```python
from build123d import *

# Parameters (mm, degrees)
SKETCH1_R           = 2.1
BOSS_EXTRUDE1_DEPTH = 200


with BuildPart() as part:
    # Sketch1 → Boss-Extrude1 (new body)
    with BuildSketch(Plane(origin=(0, 0, 0), x_dir=(1, 0, 0), z_dir=(0, 1, 0))):
        Polygon((1.8, 15.5), (1.8, 13.1), (0, 14.9), (0, 20), (5.1, 20), (6.9, 18.2), (4.5, 18.2), (4.5, 16.560660172), (7.190031555, 13.870628617), (12.839339828, 13.870628617), (15.529414018, 16.560702806), (15.529414018, 18.2), (13.1, 18.2), (14.9, 20), (25.280697212, 20), (27.080697212, 18.2), (24.470585982, 18.2), (24.470585982, 16.560702806), (27.160660172, 13.870628617), (32.809968445, 13.870628617), (35.5, 16.560660172), (35.5, 18.2), (33.1, 18.2), (34.9, 20), (40, 20), (40, 14.9), (38.2, 13.1), (38.2, 15.5), (36.560660172, 15.5), (33.870585982, 12.809925811), (33.870585982, 7.160617537), (36.560617537, 4.470585982), (38.2, 4.470585982), (38.2, 6.9), (40, 5.1), (40, 0), (34.9, 0), (33.1, 1.8), (35.499957366, 1.8), (35.499957366, 3.409925811), (32.809883176, 6.1), (27.160574903, 6.1), (24.470543348, 3.409968445), (24.470543348, 1.8), (27, 1.8), (25.2, 0), (14.9, 0), (13.1, 1.8), (15.529456652, 1.8), (15.529456652, 3.409968445), (12.839425097, 6.1), (7.190116824, 6.1), (4.500042634, 3.409925811), (4.500042634, 1.8), (6.9, 1.8), (5.1, 0), (0, 0), (0, 5.1), (1.8, 6.9), (1.8, 4.470585982), (3.439382463, 4.470585982), (6.129414018, 7.160617537), (6.129414018, 12.809925811), (3.439339828, 15.5), align=None)
        with Locations(Location((10, 10, 0), (0, 0, 270))):
            Circle(SKETCH1_R, mode=Mode.SUBTRACT)
        with Locations(Location((30, 10, 0), (0, 0, 90))):
            Circle(SKETCH1_R, mode=Mode.SUBTRACT)
        Polygon((13.900042634, 7.175345863), (13.900042634, 12.824654137), (17.029456652, 15.964292458), (17.039482597, 18.2), (22.960517403, 18.2), (22.970543348, 15.964292458), (26.099957366, 12.824654137), (26.099957366, 7.175345863), (22.970543348, 4.035707542), (22.970543348, 1.8), (17.029456652, 1.8), (17.029456652, 4.035707542), align=None, mode=Mode.SUBTRACT)
    extrude(amount=BOSS_EXTRUDE1_DEPTH)


solid = part.part
```
Model file for the job. Use its own axes, mm. A direction names the side the tool comes from. Give positions to 0.01 mm unless a question says otherwise; leave off trailing zeros. Write each loop counter-clockwise with the first axis right and the second up, starting at its lowest first coordinate (ties: lowest second). Pieces come first, ordered by that corner, then holes. Notation, with made-up numbers: (76, 15.25) - (92, 15.25) arc R27 cw to (92, 31.25) - close; hole circle Ø9 at (-17, -16.75). An arc over 180 degrees is marked (long way). One line per question, with ' | ' between items. Start each with the question number.
(1) 3-axis set-ups, long thin cutter, end or side, ignore diameter. For faces 1 (the face through (6.129, 99, -10)), 2 (the face through (10, 99, -6.1)), 3 (the face through (24.56, 98.6, -5.63)): which of +Z, -Z, +X, -X, +Y, -Y reach the whole face in a straight line?
(2) Two-plate mould, pull along Z, no slides. Class faces 4 (the face through (31.278, 98.6, -8.334)), 5 (the face through (10, 99, -13.871)), 6 (the face through (24.51, 98.6, -14.42)), 7 (the face through (25, 0, -15)): +Z half, -Z half, draft (parallel to the pull), parting line (faces both ways), or undercut.
(3) Slice it at C-C on y = 117. Give the number of separate pieces and of enclosed holes in the cut face, plus the area to 3 significant figures.
(4) Slice it at A-A on x = 10. Write the cut outline in (y, z).
(5) Slice it at B-B on z = -10. Write the cut outline in (x, y).
(6) Wall check: line 1 along X through (y, z) = (56, -16.75); line 2 along X through (y, z) = (137, -10); line 3 along Z through (x, y) = (30, 101). Give the ranges that are in metal, low to high. Write a range as from..to.
(7) Pin check, flat tips, straight feed: P1, Ø4.5, axis at y = 109.5, z = -11, coming from the -X side; P2, Ø4.5, axis at y = 109.5, z = -10.5, coming from the +X side; P3, Ø4.5, axis at x = 30, y = 112, coming from the +Z side; P4, Ø1, axis at x = 31.5, z = -15, coming from the -Y side. Stop position of each tip, or through.
Results below:
1) face 1: -X, +Y, -Y | face 2: +Z, +Y, -Y | face 3: +Y, -Y
2) face 4: undercut | face 5: -Z half | face 6: undercut | face 7: draft
3) separate pieces: 1 | enclosed holes: 3 | area: 292 mm^2
4) outline: (0, -13.87) - (200, -13.87) - (200, -12.1) - (0, -12.1) - close; (0, -7.9) - (200, -7.9) - (200, -6.1) - (0, -6.1) - close
5) outline: (6.13, 0) - (7.9, 0) - (7.9, 200) - (6.13, 200) - close; (12.1, 0) - (13.9, 0) - (13.9, 200) - (12.1, 200) - close; (26.1, 0) - (27.9, 0) - (27.9, 200) - (26.1, 200) - close; (32.1, 0) - (33.87, 0) - (33.87, 200) - (32.1, 200) - close
6) line 1: 0..4.5, 15.53..17.03, 22.97..24.47, 35.5..40 | line 2: 6.13..7.9, 12.1..13.9, 26.1..27.9, 32.1..33.87 | line 3: -13.87..-12.1, -7.9..-6.1
7) P1: x = 1.65 | P2: x = 33.87 | P3: z = -6.1 | P4: through
